For this review, take the finished solid that the model builds, in its own axes (mm). A direction names the side the tool comes from. Coordinates: 2 decimals unless noted, no trailing zeros. Loops run counter-clockwise (first coordinate to the right, second up) from the corner with the lowest first, then second, coordinate; pieces in that order, holes last. Notation, with made-up numbers: M 14.25,29.25 L 52.25,29.25 A18 ccw 52.25,43.25 Z; hole C 5,-12.5 d1. An arc over 180 degrees is marked long. Answer as a JSON object with one key per item and string values. Group by question number.
Item 1: Tool access review of faces 1 (the face through (333, 5, -200.537)), 2 (the face through (192, 5, -257.537)): name each direction out of +Z, -Z, +X, -X, +Y, -Y from which nothing blocks a thin tool from reaching the whole face with its end or side.
Item 2: Add section B-B (x = 259). State the section outline as (y, z) points.
Item 3: Add section C-C (y = 7.5). Count the separate pieces of the cut face and the enclosed holes in it, then the cut area to 3 significant figures.
Item 4: Wall thickness on L1, parallel to Z at x = 259.5, y = 7.75; L2, parallel to X at y = 2.5, z = -85; L3, parallel to X at y = 9, z = -121.5: over which ranges is each line inside the solid? List them lowest first. Write a range as from..to.
Item 5: Mouldability with a two-part tool opening along X and no side actions: class faces 3 (the face through (334, 5, -194.537)), 4 (the face through (445.616, 5, -105)), 5 (the face through (192, 5, 42.463)) as +X half, -X half, draft (parallel to the pull), parting line (faces both ways), or undercut.
Item 6: Add section A-A (x = -9). State the section outline as (y, z) points.
from build123d import *

# Parameters (mm, degrees)
SKETCH1_W           = 500
SKETCH1_H           = 300
BOSS_EXTRUDE1_DEPTH = 10
CUT_EXTRUDE1_DEPTH  = 10
CUT_EXTRUDE2_DEPTH  = 515.780562137
CUT_EXTRUDE3_DEPTH  = 515.780562137


with BuildPart() as part:
    # Sketch1 → Boss-Extrude1 (new body)
    with BuildSketch(Plane(origin=(0, 0, 0), x_dir=(1, 0, 0), z_dir=(0, 1, 0))):
        with Locations((195.615833125, 107.53748547)):
            Rectangle(SKETCH1_W, SKETCH1_H)
    extrude(amount=BOSS_EXTRUDE1_DEPTH)

    # Sketch2 → Cut-Extrude1 (cut)
    with BuildSketch(Plane(origin=(0, 10, 0), x_dir=(1, 0, 0), z_dir=(0, 1, 0))):
        with BuildLine():
            Line((208.615833125, 168.829709188), (208.615833125, 122.242622587))
            ThreePointArc((208.615833125, 122.242622587), (205.615833125, 119.242622587), (202.615833125, 122.242622587))
            Line((202.615833125, 122.242622587), (202.615833125, 168.829709188))
            ThreePointArc((202.615833125, 168.829709188), (205.615833125, 171.829709188), (208.615833125, 168.829709188))
        make_face()
        with BuildLine():
            Line((208.615833125, 46.245261752), (208.615833125, 92.832348352))
            ThreePointArc((208.615833125, 92.832348352), (205.615833125, 95.832348352), (202.615833125, 92.832348352))
            Line((202.615833125, 92.832348352), (202.615833125, 46.245261752))
            ThreePointArc((202.615833125, 46.245261752), (205.615833125, 43.245261752), (208.615833125, 46.245261752))
        make_face()
        with BuildLine():
            Line((356.908056843, 194.53748547), (310.320970243, 194.53748547))
            ThreePointArc((310.320970243, 194.53748547), (307.320970243, 197.53748547), (310.320970243, 200.53748547))
            Line((310.320970243, 200.53748547), (356.908056843, 200.53748547))
            ThreePointArc((356.908056843, 200.53748547), (359.908056843, 197.53748547), (356.908056843, 194.53748547))
        make_face()
        with BuildLine():
            Line((234.323609407, 194.53748547), (280.910696008, 194.53748547))
            ThreePointArc((280.910696008, 194.53748547), (283.910696008, 197.53748547), (280.910696008, 200.53748547))
            Line((280.910696008, 200.53748547), (234.323609407, 200.53748547))
            ThreePointArc((234.323609407, 200.53748547), (231.323609407, 197.53748547), (234.323609407, 194.53748547))
        make_face()
        with BuildLine():
            Line((382.615833125, 46.245261752), (382.615833125, 92.832348352))
            ThreePointArc((382.615833125, 92.832348352), (385.615833125, 95.832348352), (388.615833125, 92.832348352))
            Line((388.615833125, 92.832348352), (388.615833125, 46.245261752))
            ThreePointArc((388.615833125, 46.245261752), (385.615833125, 43.245261752), (382.615833125, 46.245261752))
        make_face()
        with BuildLine():
            Line((382.615833125, 168.829709188), (382.615833125, 122.242622587))
            ThreePointArc((382.615833125, 122.242622587), (385.615833125, 119.242622587), (388.615833125, 122.242622587))
            Line((388.615833125, 122.242622587), (388.615833125, 168.829709188))
            ThreePointArc((388.615833125, 168.829709188), (385.615833125, 171.829709188), (382.615833125, 168.829709188))
        make_face()
        with BuildLine():
            Line((234.323609407, 20.53748547), (280.910696008, 20.53748547))
            ThreePointArc((280.910696008, 20.53748547), (283.910696008, 17.53748547), (280.910696008, 14.53748547))
            Line((280.910696008, 14.53748547), (234.323609407, 14.53748547))
            ThreePointArc((234.323609407, 14.53748547), (231.323609407, 17.53748547), (234.323609407, 20.53748547))
        make_face()
        with BuildLine():
            Line((356.908056843, 20.53748547), (310.320970243, 20.53748547))
            ThreePointArc((310.320970243, 20.53748547), (307.320970243, 17.53748547), (310.320970243, 14.53748547))
            Line((310.320970243, 14.53748547), (356.908056843, 14.53748547))
            ThreePointArc((356.908056843, 14.53748547), (359.908056843, 17.53748547), (356.908056843, 20.53748547))
        make_face()
    extrude(amount=-CUT_EXTRUDE1_DEPTH, mode=Mode.SUBTRACT)

    # Sketch6 → Cut-Extrude2 (cut, through all)
    with BuildSketch(Plane(origin=(0, 10, 0), x_dir=(1, 0, 0), z_dir=(0, 1, 0))):
        with BuildLine():
            Line((-43.900749025, 110.53748547), (118.112557876, 110.53748547))
            ThreePointArc((118.112557876, 110.53748547), (121.112557876, 107.53748547), (118.112557876, 104.53748547))
            Line((118.112557876, 104.53748547), (-43.900749025, 104.53748547))
            ThreePointArc((-43.900749025, 104.53748547), (-46.900749025, 107.53748547), (-43.900749025, 110.53748547))
        make_face()
    extrude(amount=-CUT_EXTRUDE2_DEPTH, mode=Mode.SUBTRACT)

    # Sketch7 → Cut-Extrude3 (cut, through all)
    with BuildSketch(Plane(origin=(0, 10, 0), x_dir=(1, 0, 0), z_dir=(0, 1, 0))):
        with BuildLine():
            Line((292.615833125, 110.53748547), (292.615833125, 157.53748547))
            ThreePointArc((292.615833125, 157.53748547), (295.615833125, 160.53748547), (298.615833125, 157.53748547))
            Line((298.615833125, 157.53748547), (298.615833125, 110.53748547))
            Line((298.615833125, 110.53748547), (350.356251663, 110.53748547))
            ThreePointArc((350.356251663, 110.53748547), (353.356251663, 107.53748547), (350.356251663, 104.53748547))
            Line((350.356251663, 104.53748547), (298.615833125, 104.53748547))
            Line((298.615833125, 104.53748547), (298.615833125, 57.53748547))
            ThreePointArc((298.615833125, 57.53748547), (295.615833125, 54.53748547), (292.615833125, 57.53748547))
            Line((292.615833125, 57.53748547), (292.615833125, 104.53748547))
            Line((292.615833125, 104.53748547), (240.875414588, 104.53748547))
            ThreePointArc((240.875414588, 104.53748547), (237.875414588, 107.53748547), (240.875414588, 110.53748547))
            Line((240.875414588, 110.53748547), (292.615833125, 110.53748547))
        make_face()
    extrude(amount=-CUT_EXTRUDE3_DEPTH, mode=Mode.SUBTRACT)


solid = part.part
From the geometry:
{
 "1": {"face 1": "+Y, -Y", "face 2": "-Z, +X, -X, +Y, -Y"},
 "2": {"outline": "M 0,-257.54 L 10,-257.54 L 10,-200.54 L 0,-200.54 Z; M 0,-194.54 L 10,-194.54 L 10,-110.54 L 0,-110.54 Z; M 0,-104.54 L 10,-104.54 L 10,-20.54 L 0,-20.54 Z; M 0,-14.54 L 10,-14.54 L 10,42.46 L 0,42.46 Z"},
 "3": {"separate pieces": "1", "enclosed holes": "10", "area": "145,000 mm²"},
 "4": {"L1": "z = -257.54..-200.54, -194.54..-110.54, -104.54..-20.54, -14.54..42.46", "L2": "x = -54.38..202.62, 208.62..292.62, 298.62..382.62, 388.62..445.62", "L3": "x = -54.38..202.71, 208.52..292.62, 298.62..382.71, 388.52..445.62"},
 "5": {"face 3": "undercut", "face 4": "+X half", "face 5": "draft"},
 "6": {"outline": "M 0,-257.54 L 10,-257.54 L 10,-110.54 L 0,-110.54 Z; M 0,-104.54 L 10,-104.54 L 10,42.46 L 0,42.46 Z"}
}
